The model under review builds one solid part; all positions refer to its coordinate system, in mm. Face numbers are marked on the shaded views. A direction names the side the tool comes from. Give positions to 0.01 mm unless a question says otherwise; leave off trailing zeros. Loops run counter-clockwise (first coordinate to the right, second up) from the corner with the lowest first, then second, coordinate; pieces in that order, holes last. Notation, with made-up numbers: M -23.5,82 L -14.5,82 A13 cw -14.5,97 Z; hole C 82,3.25 d9. An arc over 180 degrees is marked long. Put each result on its own line as item: value. Start each with the question number.
from build123d import *

# Parameters (mm, degrees)
BOSS_EXTRUDE1_DEPTH     = 100
FILLET1_R               = 5
FILLET2_R               = 5
FILLET3_R               = 20
FILLET4_R               = 20
SKETCH5_R               = 15
CUT_EXTRUDE1_DEPTH      = 208.498638182
SKETCH16_R              = 15
CUT_EXTRUDE5_DEPTH      = 208.498638182
CUT_EXTRUDE8_DEPTH      = 208.498638182
CUT_EXTRUDE8_DEPTH_BACK = 208.498638182


with BuildPart() as part:
    # Sketch4 → Boss-Extrude1 (new body)
    with BuildSketch(Plane.XY):
        with BuildLine():
            Line((-40, -60), (-30, -60))
            Line((-30, -60), (0, -60))
            Line((0, -60), (30, -60))
            Line((30, -60), (40, -60))
            Line((40, -60), (40, 164.983908243))
            ThreePointArc((40, 164.983908243), (39.979276225, 164.991956207), (39.958550831, 165))
            ThreePointArc((39.958550831, 165), (0, 172.480244803), (-39.958550831, 165))
            ThreePointArc((-39.958550831, 165), (-39.979276225, 164.991956207), (-40, 164.983908243))
            Line((-40, 164.983908243), (-40, -60))
        make_face()
        Polygon((-30, -60), (-30, -105), (0, -105), (30, -105), (30, -60), (0, -60), align=None)
        Polygon((57.5, -120), (-57.5, -120), (-57.5, -150), (0, -150), (57.5, -150), align=None)
        Polygon((0, -105), (-30, -105), (-30, -120), (30, -120), (30, -105), align=None)
    extrude(amount=BOSS_EXTRUDE1_DEPTH)

    # Fillet1
    fillet1_edges = [part.edges().sort_by_distance(p)[0] for p in [
        (-30, -60, 50),
    ]]
    fillet(fillet1_edges, radius=FILLET1_R)

    # Fillet2
    fillet2_edges = [part.edges().sort_by_distance(p)[0] for p in [
        (30, -60, 50),
    ]]
    fillet(fillet2_edges, radius=FILLET2_R)

    # Fillet3
    fillet3_edges = [part.edges().sort_by_distance(p)[0] for p in [
        (-30, -120, 50),
    ]]
    fillet(fillet3_edges, radius=FILLET3_R)

    # Fillet4
    fillet4_edges = [part.edges().sort_by_distance(p)[0] for p in [
        (30, -120, 50),
    ]]
    fillet(fillet4_edges, radius=FILLET4_R)

    # Sketch5 → Cut-Extrude1 (cut, through all)
    with BuildSketch(Plane.XY.offset(100)):
        with Locations((0, 120)):
            Circle(SKETCH5_R)
    extrude(amount=-CUT_EXTRUDE1_DEPTH, mode=Mode.SUBTRACT)

    # Sketch16 → Cut-Extrude5 (cut, through all)
    with BuildSketch(Plane.XY.offset(100)):
        with Locations((0, -30)):
            Circle(SKETCH16_R)
    extrude(amount=-CUT_EXTRUDE5_DEPTH, mode=Mode.SUBTRACT)

    # Sketch19 → Cut-Extrude8 (cut, two sides: drawn at the far end of the back side and taken through both)
    with BuildSketch(Plane(origin=(0, 0, 0), x_dir=(0, 0, -1), z_dir=(1, 0, 0)).offset(-CUT_EXTRUDE8_DEPTH_BACK)):
        with BuildLine():
            Line((-50, 93), (-100, 93))
            Line((-100, 93), (-100, -3))
            Line((-100, -3), (-50, -3))
            ThreePointArc((-50, -3), (-2, 45), (-50, 93))
        make_face()
    extrude(amount=CUT_EXTRUDE8_DEPTH + CUT_EXTRUDE8_DEPTH_BACK, mode=Mode.SUBTRACT)


solid = part.part
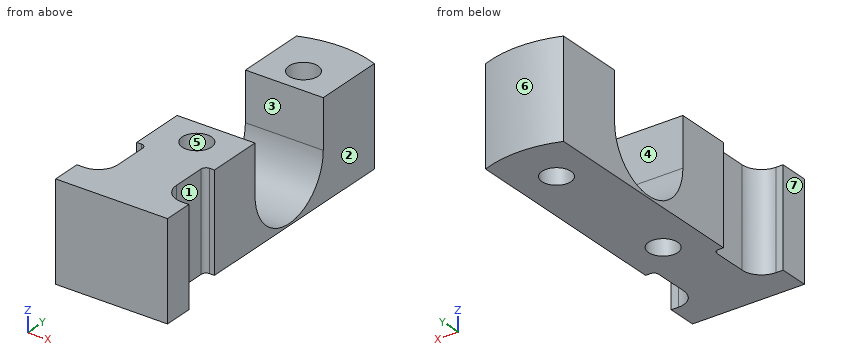
(1) For the marked faces 1, 2 and 3, list the 3-axis set-ups (+Z, -Z, +X, -X, +Y, -Y) from which the entire face can be reached by the end or side of a thin tool; tool diameter is ignored.
(2) We need section D-D, the plane z = 39. Write out the cut boundary in (x, y), plus the area to 3 significant figures.
(3) We need section C-C, the plane x = 8. Write out the cut boundary in (y, z), plus the area to 3 significant figures.
(4) Insertion check: pin 1 (6 mm diameter, centred on x = 21.5, y = -105.5, fed in from -Z); pin 2 (6 mm diameter, centred on x = 55, z = 51.5, fed in from +Y); pin 3 (5 mm diameter, centred on y = -51.5, z = 77.5, fed in from +X); pin 4 (4 mm diameter, centred on y = -103, z = 87.5, fed in from -X). Each pin has a flat end and moves straight along its axis. Give the tip position at first contact, or say it passes through.
(5) We need section A-A, the plane z = 69. Write out the cut boundary in (x, y), plus the area to 3 significant figures.
(6) Draft analysis for pull direction Y (two halves, no side actions). For the marked faces 4, 5, 6 and 7, state which applies: +Y half, -Y half, draft (parallel to the pull), parting line (faces both ways), or undercut.
(7) We need section B-B, the plane y = -30. Write out the cut boundary in (x, z), plus the area to 3 significant figures.
(8) To check wall thickness, follow L1, parallel to Y at x = 0, z = 55; L2, parallel to Y at x = 35, z = 8.5; L3, parallel to X at y = -49, z = 85.5. State the ranges of each line that lie inside material, in increasing order. Write a range as [from, to].
Check sheet entries:
1. face 1: +Z, -Z, +X
1. face 2: +Z, -Z, +X, +Y
1. face 3: +Z, +X, -X
2. outline: M -57.5,-150 L 57.5,-150 L 57.5,-120 L 50,-120 A20 cw 30,-100 L 30,-65 A5 cw 35,-60 L 40,-60 L 40,-1.72 L -40,-1.72 L -40,-60 L -35,-60 A5 cw -30,-65 L -30,-100 A20 cw -50,-120 L -57.5,-120 Z; M -40,91.72 L 40,91.72 L 40,164.98 A110.47 ccw 39.96,165 A110.47 ccw -39.96,165 A110.47 ccw -40,164.98 Z; hole C 0,-30 d30; hole C 0,120 d30
2. area: 16,700 mm²
3. outline: M -150,0 L -42.69,0 L -42.69,100 L -150,100 Z; M -17.31,0 L 107.31,0 L 107.31,100 L 93,100 L 93,50 A48 cw -3,50 L -3,100 L -17.31,100 Z; M 132.69,0 L 172.19,0 L 172.19,100 L 132.69,100 Z
3. area: 18,700 mm²
4. pin 1: stops at z = 0
4. pin 2: stops at y = -120
4. pin 3: stops at x = 40
4. pin 4: stops at x = -30.64
5. outline: M -57.5,-150 L 57.5,-150 L 57.5,-120 L 50,-120 A20 cw 30,-100 L 30,-65 A5 cw 35,-60 L 40,-60 L 40,-3 L -40,-3 L -40,-60 L -35,-60 A5 cw -30,-65 L -30,-100 A20 cw -50,-120 L -57.5,-120 Z; M -40,93 L 40,93 L 40,164.98 A110.47 ccw 39.96,165 A110.47 ccw -39.96,165 A110.47 ccw -40,164.98 Z; hole C 0,-30 d30; hole C 0,120 d30
5. area: 16,500 mm²
6. face 4: undercut
6. face 5: undercut
6. face 6: +Y half
6. face 7: draft
7. outline: M -40,0 L -15,0 L -15,100 L -40,100 Z; M 15,0 L 40,0 L 40,100 L 15,100 Z
7. area: 5,000 mm²
8. L1: y = [-150, -45], [-15, -3], [93, 105], [135, 172.48]
8. L2: y = [-150, -113.23], [-60, 20.88], [69.12, 166.79]
8. L3: x = [-40, 40]
